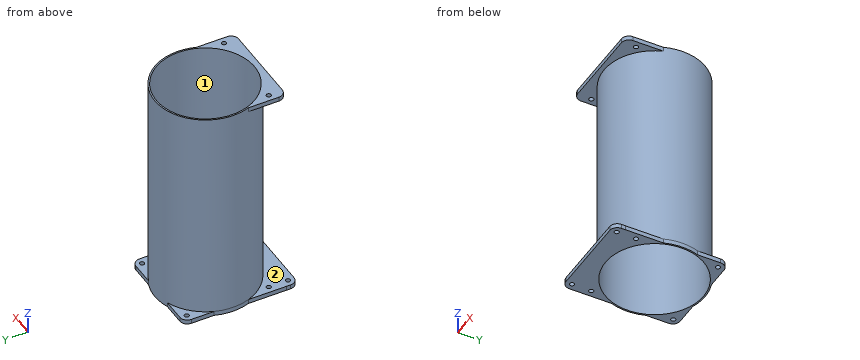
from build123d import *

# Parameters (mm, degrees)
SKETCH_2_R            = 1.5499999999999978
SKETCH_2_R_2          = 1.5500000000187404
SKETCH_2_R_3          = 33.000000000018005
SKETCH_2_R_4          = 1.5500000000180028
EXTRUDE_1_DEPTH       = 3
EXTRUDE_START         = 3
EXTRUDE_2_OUTLINE_R   = 34
EXTRUDE_2_OUTLINE_R_2 = 33
EXTRUDE_2_DEPTH       = 147
EXTRUDE_START_2       = -3
SKETCH_5_R            = 1.5499999999999978
SKETCH_5_R_2          = 1.5500000000187402
EXTRUDE_3_DEPTH       = 3


# Read off the part's stored shape, not the designer's step: 凸台-拉伸2
with BuildPart() as part:
    # 草图2 → 凸台-拉伸1 (new body)
    with BuildSketch(Plane.XY.offset(50)):
        with BuildLine():
            Line((-31.98646774923986, 34.973103667177796), (-31.986467749238788, 9.470000000000049))
            Line((-31.986467749238788, 9.47000000000005), (-31.99138785319973, 6.608597351179577))
            ThreePointArc((-31.99138785319973, 6.608597351179577), (-30.529967467729293, 3.0675070244866425), (-26.991395244649887, 1.5999999999999854))
            Line((-26.991395244649887, 1.5999999999999854), (26.99139524464973, 1.6000000000000048))
            ThreePointArc((26.99139524464973, 1.600000000000005), (30.529967467729193, 3.067507024486723), (31.99138785319957, 6.6085973511797595))
            Line((31.99138785319957, 6.6085973511797595), (31.98646774923853, 9.470000000001768))
            Line((31.98646774923853, 9.470000000001768), (31.986467749238717, 34.9731036671784))
            ThreePointArc((31.986467749239328, 34.97310366717818), (34.000000000018005, 46.499849995960744), (31.986467749239164, 58.026596324743274))
            Line((31.986467749238994, 58.02659632474322), (31.98646774923853, 73.4863177451979))
            ThreePointArc((31.986467749238525, 73.4863177451979), (30.52200165517117, 77.02185165113154), (26.986467749237562, 78.486317745199))
            Line((26.986467749237562, 78.486317745199), (11.526746328783656, 78.48631774519934))
            ThreePointArc((11.526746328783661, 78.48631774519934), (1.3678e-13, 80.49984999597851), (-11.5267463287834, 78.48631774519944))
            Line((-11.526746328783396, 78.48631774519944), (-26.98646774923796, 78.48631774520034))
            ThreePointArc((-26.98646774923796, 78.48631774520034), (-30.52200165517142, 77.02185165113266), (-31.98646774923918, 73.48631774519924))
            Line((-31.986467749239182, 73.48631774519924), (-31.986467749239175, 58.02659632474571))
            ThreePointArc((-31.986467749239328, 58.026596324742826), (-34.000000000018005, 46.4998499959604), (-31.986467749239267, 34.973103667178016))
        make_face()
        with Locations((-27.577164466275363, 5.922685529685147)):
            Circle(SKETCH_2_R, mode=Mode.SUBTRACT)
        with Locations((-27.577164466275352, 18.922685529685147)):
            Circle(SKETCH_2_R_2, mode=Mode.SUBTRACT)
        with Locations((27.57716446627534, 5.92268552968515)):
            Circle(SKETCH_2_R, mode=Mode.SUBTRACT)
        with Locations((27.577164466275352, 18.922685529685147)):
            Circle(SKETCH_2_R_2, mode=Mode.SUBTRACT)
        with Locations((0, 46.4998499959605)):
            Circle(SKETCH_2_R_3, mode=Mode.SUBTRACT)
        with Locations((-27.577164466275352, 74.07701446223585)):
            Circle(SKETCH_2_R_4, mode=Mode.SUBTRACT)
        with Locations((27.577164466275352, 74.07701446223585)):
            Circle(SKETCH_2_R_4, mode=Mode.SUBTRACT)
    extrude(amount=EXTRUDE_1_DEPTH)

    # 凸台-拉伸2 outline → 凸台-拉伸2 (add)
    with BuildSketch(Plane.XY.offset(50).offset(EXTRUDE_START)):
        with Locations((0, 46.499849996)):
            Circle(EXTRUDE_2_OUTLINE_R)
        with Locations((0, 46.499849996)):
            Circle(EXTRUDE_2_OUTLINE_R_2, mode=Mode.SUBTRACT)
    extrude(amount=EXTRUDE_2_DEPTH)

    # 草图5 → 凸台-拉伸3 (add)
    # profile 1 of 3: a face of its own
    with BuildSketch(Plane.XY.offset(200).offset(EXTRUDE_START_2)):
        with Locations((27.57716446627534, 5.92268552968515)):
            Circle(SKETCH_5_R)
    # profile 2 of 3: a face of its own
    with BuildSketch(Plane.XY.offset(200).offset(EXTRUDE_START_2)):
        with Locations((-27.577164466275363, 5.922685529685147)):
            Circle(SKETCH_5_R)
    # profile 3 of 3: a face of its own
    with BuildSketch(Plane.XY.offset(200).offset(EXTRUDE_START_2)):
        with BuildLine():
            Line((31.986467749238557, 14.470000000001733), (31.986467749238717, 34.9731036671784))
            ThreePointArc((31.986467749238717, 34.9731036671784), (6.9664e-13, 12.499849995942498), (-31.98646774923986, 34.973103667177796))
            Line((-31.98646774923986, 34.973103667177796), (-31.986467749238994, 14.470000000001559))
            ThreePointArc((-31.986467749238994, 14.470000000001559), (-30.522001655171657, 10.934466094068965), (-26.986467749239004, 9.470000000001766))
            Line((-26.986467749239004, 9.470000000001766), (26.986467749238557, 9.470000000001766))
            ThreePointArc((26.986467749238557, 9.470000000001766), (30.52200165517128, 10.93446609406902), (31.986467749238557, 14.470000000001733))
        make_face()
        with Locations((27.577164466275352, 18.922685529685147)):
            Circle(SKETCH_5_R_2, mode=Mode.SUBTRACT)
        with Locations((-27.577164466275352, 18.922685529685147)):
            Circle(SKETCH_5_R_2, mode=Mode.SUBTRACT)
    extrude(amount=EXTRUDE_3_DEPTH)


with BuildPart() as extrude_3_kept_piece:
    # of the separate pieces the step leaves, the one the design keeps (extrude_3_pieces_kept)
    add(part.part.solids().sort_by_distance((-31.986467749, 58.026596325, 50))[0])


solid = extrude_3_kept_piece.part
Verification items for the finished model (mm, model axes). Face numbers are marked on the shaded views. Give positions to 0.01 mm unless a question says otherwise; leave off trailing zeros. Loops run counter-clockwise (first coordinate to the right, second up) from the corner with the lowest first, then second, coordinate; pieces in that order, holes last. Notation, with made-up numbers: (33.25, -37.75) - (68.25, -37.75) arc R14 ccw to (68.25, -22.75) - close; hole circle Ø3 at (83.5, 59.5). An arc over 180 degrees is marked (long way). Write item = value, one per line. Start each with the question number.
Q1. Thickness scan on line 1 (Z direction, x = 21, y = 11); line 2 (X direction, y = 55, z = 65); line 3 (X direction, y = 24, z = 161). Record the ranges inside material, lowest first.
Q2. Cross-section at A-A, the plane x = 0. Enter the section's corners in (y, z), and give its area (3 significant figures).
Q3. Depth check by flat-ended pin: P1, Ø0.9, axis at y = 21.5, z = 199, coming from the +X side; P2, Ø1.5, axis at x = -18, z = 51.5, coming from the +Y side; P3, Ø1.5, axis at x = 3.5, z = 157, coming from the +Y side; P4, Ø2.5, axis at x = 27.58, y = 18.92, coming from the -Z side. Enter the tip coordinate at first touch or a pass-through.
Q4. Cross-section at D-D, the plane x = -23. Enter the section's corners in (y, z).
Q5. Cross-section at C-C, the plane z = 115. Enter the section's corners in (x, y), and give its area (3 significant figures).
Q6. Cross-section at B-B, the plane y = 24. Enter the section's corners in (x, z).
Q7. Mould release check, pull along X, two halves, no side actions. Record for the marked faces 1 and 2: released by +X, released by -X, zero draft, split by the parting line, or undercut.
Answer key:
q1.line_1 = 50 to 53, 197 to 200
q1.line_2 = -32.92 to -31.89, 31.89 to 32.92
q1.line_3 = -25.49 to -24.14, 24.14 to 25.49
q2.outline = (1.6, 50) - (13.5, 50) - (13.5, 200) - (9.47, 200) - (9.47, 197) - (12.5, 197) - (12.5, 53) - (1.6, 53) - close; (79.5, 50) - (80.5, 50) - (80.5, 200) - (79.5, 200) - close
q2.area = 342 mm^2
q3.P1 = 31.99
q3.P2 = 78.49
q3.P3 = 80.39
q3.P4 = through
q4.outline = (1.6, 50) - (22.84, 50) - (22.84, 200) - (9.47, 200) - (9.47, 197) - (21.46, 197) - (21.46, 53) - (1.6, 53) - close; (70.16, 50) - (78.49, 50) - (78.49, 53) - (71.54, 53) - (71.54, 200) - (70.16, 200) - close
q5.outline = circle Ø68 at (0, 46.5); hole circle Ø66 at (0, 46.5)
q5.area = 210 mm^2
q6.outline = (-31.99, 50) - (-24.14, 50) - (-24.14, 200) - (-31.99, 200) - (-31.99, 197) - (-25.49, 197) - (-25.49, 53) - (-31.99, 53) - close; (24.14, 50) - (31.99, 50) - (31.99, 53) - (25.49, 53) - (25.49, 197) - (31.99, 197) - (31.99, 200) - (24.14, 200) - close
q7.face_1 = undercut
q7.face_2 = zero draft
